Autodesk Fusion 360 part; units mm, degrees
sketch "Sketch1" plane through (0, 0, 0) normal (0, 0, 1) x (1, 0, 0)
  line L0 (30, -12.5) -> (-30, -12.5)
  line L1 (-30, -12.5) -> (-30, 12.5)
  line L2 (-30, 12.5) -> (30, 12.5)
  line L3 (30, 12.5) -> (30, -12.5)
  line L4 (30, -12.5) -> (-30, 12.5) construction
  line L5 (-30, -12.5) -> (30, 12.5) construction
  circle A0 centre (-15, -7.5) radius 1.5
  circle A1 centre (4, -7.5) radius 1.5
  line L6 (-27.625, 8.5) -> (-27.625, -1.5)
  arc A2 (-27.625, -1.5) -> (-22.375, -1.5) centre (-25, -1.5) ccw
  line L7 (-22.375, -1.5) -> (-22.375, 8.5)
  arc A3 (-22.375, 8.5) -> (-27.625, 8.5) centre (-25, 8.5) ccw
  line L8 (-25, 8.5) -> (-25, -1.5) construction
  line L9 (27.625, -1.5) -> (27.625, 8.5)
  arc A4 (27.625, 8.5) -> (22.375, 8.5) centre (25, 8.5) ccw
  line L10 (22.375, 8.5) -> (22.375, -1.5)
  arc A5 (22.375, -1.5) -> (27.625, -1.5) centre (25, -1.5) ccw
  line L11 (25, -1.5) -> (25, 8.5) construction
  dimension "d1" = 60
  dimension "d2" = 25
  dimension "d3" = 3
  dimension "d4" = 3
  dimension "d5" = 19
  dimension "d6" = 5
  dimension "d7" = 5
  dimension "d8" = 15
  dimension "d9" = 5.25
  dimension "d10" = 5.25
  dimension "d11" = 5
  dimension "d12" = 5
  dimension "d15" = 4
  dimension "d16" = 4
  dimension "d17" = 10
  dimension "d18" = 10
extrude "Extrude1" add sketch "Sketch1" along normal blind 5
equation "d7 = d6"
equation "d10 = d9"
equation "d12 = d11"
equation "d16 = d15"
equation "d18 = d17"
Geometry check sheet. Reference: the model listing, model coordinates, mm. A direction names the side the tool comes from. Round coordinates to 2 decimals unless told otherwise and drop trailing zeros. Loops run counter-clockwise (first coordinate to the right, second up) from the corner with the lowest first, then second, coordinate; pieces in that order, holes last. Notation, with made-up numbers: (-11, -18) - (1, -18) arc R22 cw to (1, -9) - close; hole circle Ø5 at (7, 81). An arc over 180 degrees is marked (long way). Use a Markdown table: item, result.
Q1. Access from +Z, -Z, +X, -X, +Y, -Y to the whole of each face (thin tool, end or side, straight path). Record for faces 1 (the flat face through (-27.625, 4, 2)), 2 (the flat face through (0, -12.5, 2)).
Solutions:
| item | result |
|---|---|
| face 1 | +Z, -Z |
| face 2 | +Z, -Z, +X, -X, -Y |
Q2. Cross-section at A-A on y = 1. Record the cut outline in (x, z) (3 decimals).
Solutions:
| item | result |
|---|---|
| outline | (-30, 0) - (-27.625, 0) - (-27.625, 5) - (-30, 5) - close; (-22.375, 0) - (22.375, 0) - (22.375, 5) - (-22.375, 5) - close; (27.625, 0) - (30, 0) - (30, 5) - (27.625, 5) - close |
Q3. Cross-section at D-D on x = -25. Record the cut outline in (y, z) (3 decimals).
Solutions:
| item | result |
|---|---|
| outline | (-12.5, 0) - (-4.125, 0) - (-4.125, 5) - (-12.5, 5) - close; (11.125, 0) - (12.5, 0) - (12.5, 5) - (11.125, 5) - close |
Q4. Draft check along Y on faces 3 (the flat face through (0, 0, 5)), 4 (the cylindrical face through (-25.058, 11.124, 2.465)), 5 (the flat face through (0, 12.5, 2)). Enter one of: released by +Y, released by -Y, zero draft, split by the parting line, or undercut.
Solutions:
| item | result |
|---|---|
| face 3 | zero draft |
| face 4 | undercut |
| face 5 | released by +Y |
Q5. Cross-section at B-B on z = 1.95. Record the cut outline in (x, y) (3 decimals).
Solutions:
| item | result |
|---|---|
| outline | (-30, -12.5) - (30, -12.5) - (30, 12.5) - (-30, 12.5) - close; hole (-27.625, -1.5) arc R2.625 ccw to (-22.375, -1.5) - (-22.375, 8.5) arc R2.625 ccw to (-27.625, 8.5) - close; hole circle Ø3 at (-15, -7.5); hole circle Ø3 at (4, -7.5); hole (22.375, -1.5) arc R2.625 ccw to (27.625, -1.5) - (27.625, 8.5) arc R2.625 ccw to (22.375, 8.5) - close |
Q6. Material ranges on line 1 (X direction, y = 6.25, z = 1.75) (3 decimals); line 2 (Y direction, x = -15, z = 2.15); line 3 (X direction, y = 10, z = 2.35), recorded low to high.
Solutions:
| item | result |
|---|---|
| line 1 | x = -30 to -27.625, -22.375 to 22.375, 27.625 to 30 |
| line 2 | y = -12.5 to -9, -6 to 12.5 |
| line 3 | x = -30 to -27.15, -22.85 to 22.85, 27.15 to 30 |
Q7. Cross-section at C-C on x = 4. Record the cut outline in (y, z), plus the area to 3 significant figures.
Solutions:
| item | result |
|---|---|
| outline | (-12.5, 0) - (-9, 0) - (-9, 5) - (-12.5, 5) - close; (-6, 0) - (12.5, 0) - (12.5, 5) - (-6, 5) - close |
| area | 110 mm2 |
Q8. Go/stop test with a flat-tipped pin: P1, Ø1.8, axis at x = -15, y = -7.5, coming from the -Z side. Record where the tip stops, or that it passes through.
Solutions:
| item | result |
|---|---|
| P1 | passes through |
